The model under review builds one solid part; all positions refer to its coordinate system, in mm. Face numbers are marked on the shaded views. A direction names the side the tool comes from. Give positions to 0.01 mm unless a question says otherwise; leave off trailing zeros. Order: outer loops, then holes, each group sorted by start corner. A loop starts at its lowest first (then second) coordinate and runs counter-clockwise, first axis right, second up.
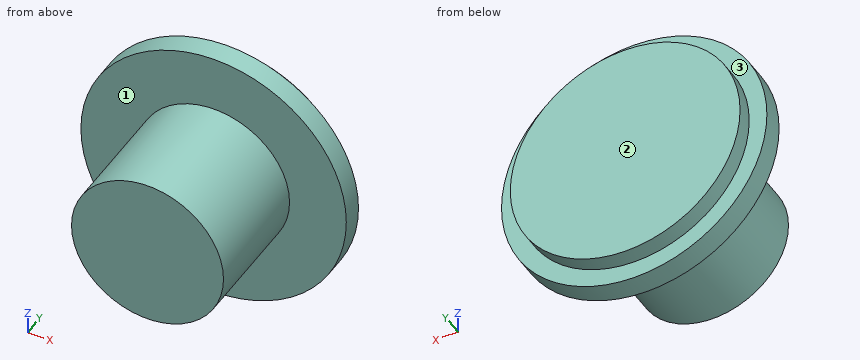
```python
from build123d import *

# Parameters (mm, degrees)
F3_R     = 311.825
F4_DEPTH = 45
F5_R     = 206.25
F6_DEPTH = 385
F7_R     = 360.125
F8_DEPTH = 60


with BuildPart() as f4:
    # F3 (on Front) → F4 (new body)
    with BuildSketch(Plane.XZ):
        with Locations((0.15, 0)):
            Circle(F3_R)
    extrude(amount=-F4_DEPTH)

    # F5 (on face) → F6 (join)
    with BuildSketch(Plane.XZ):
        with Locations((0.3, 0)):
            Circle(F5_R)
    extrude(amount=F6_DEPTH)

    # F7 (on face) → F8 (join)
    with BuildSketch(Plane.XZ):
        with Locations((0.45, 0)):
            Circle(F7_R)
    extrude(amount=F8_DEPTH)


solid = f4.part
```
Item 1: Take a section at A-A (z = 0). Give the boundary of the cut face in (x, y) (3 decimals).
Values found:
outline: (-359.675, -60) - (-205.95, -60) - (-205.95, -385) - (206.55, -385) - (206.55, -60) - (360.575, -60) - (360.575, 0) - (311.975, 0) - (311.975, 45) - (-311.675, 45) - (-311.675, 0) - (-359.675, 0) - close
Item 2: For the marked faces 1, 2 and 3, list the 3-axis set-ups (+Z, -Z, +X, -X, +Y, -Y) from which the entire face can be reached by the end or side of a thin tool; tool diameter is ignored.
Values found:
face 1: -Y
face 2: +Z, -Z, +X, -X, +Y
face 3: +Y
Item 3: For line 1 (Y direction, x = -192.5, z = 131.5); line 2 (Y direction, x = -30.5, z = -313); line 3 (Z direction, x = 142, y = -84.5), list the stretches that pass through material, from the lowest coordinate up.
Values found:
line 1: y = -60 to 45
line 2: y = -60 to 0
line 3: z = -149.87 to 149.87
Item 4: Take a section at D-D (z = -272.5). Give the boundary of the cut face in (x, y), and give its area (3 significant figures).
Values found:
outline: (-234.99, -60) - (235.89, -60) - (235.89, 0) - (151.74, 0) - (151.74, 45) - (-151.44, 45) - (-151.44, 0) - (-234.99, 0) - close
area: 41,900 mm2
Item 5: Clearance check with flat-ended pins moving along their axes: pin 1 Ø1 at (y, z) = (-51.5, 91.5) entering from -X; pin 2 Ø8 at (x, y) = (-213.5, -113.5) entering from +Z; pin 3 Ø1 at (x, z) = (-136.5, -195.5) entering from -Y; pin 4 Ø10 at (x, y) = (68.5, -129.5) entering from +Z. State where each tip first meets the part, or that it passes through.
Values found:
pin 1: stops at x = -347.99
pin 2: passes through
pin 3: stops at y = -60
pin 4: stops at z = 196.33
Item 6: Take a section at C-C (y = -200.5). Give the boundary of the cut face in (x, z), and give its area (3 significant figures).
Values found:
outline: circle Ø412.5 at (0.3, 0)
area: 134,000 mm2
Item 7: Take a section at B-B (x = 6.5). Give the boundary of the cut face in (y, z), and give its area (3 significant figures).
Values found:
outline: (-385, -206.16) - (-60, -206.16) - (-60, -360.07) - (0, -360.07) - (0, -311.76) - (45, -311.76) - (45, 311.76) - (0, 311.76) - (0, 360.07) - (-60, 360.07) - (-60, 206.16) - (-385, 206.16) - close
area: 205,000 mm2
